The listing builds one solid part. Answer for the finished solid, in the listing's coordinates (mm). A direction names the side the tool comes from. Give positions to 0.01 mm unless a question says otherwise; leave off trailing zeros. Loops run counter-clockwise (first coordinate to the right, second up) from the corner with the lowest first, then second, coordinate; pieces in that order, holes last. Notation, with made-up numbers: M 16.5,27.5 L 27.5,27.5 A17 cw 27.5,38.5 Z; hole C 7,54.25 d7. An arc over 180 degrees is marked long. Return JSON: item names as keys, results as strings.
from build123d import *

# Parameters (mm, degrees)
SKIZZE1_W                            = 42
SKIZZE1_H                            = 25
AUFSATZ_LINEAR_AUSTRAGEN1_DEPTH      = 25
SKIZZE2_W                            = 21
SKIZZE2_H                            = 21
SCHNITT_LINEAR_AUSTRAGEN1_DEPTH      = 43
SCHNITT_LINEAR_AUSTRAGEN2_DEPTH      = 5
SKIZZE4_W                            = 8.8
SKIZZE4_H                            = 21.963947762
AUFSATZ_LINEAR_AUSTRAGEN2_DEPTH      = 21
SCHNITT_LINEAR_AUSTRAGEN3_REACH      = 27
SCHNITT_LINEAR_AUSTRAGEN4_DEPTH      = 5
DURCHGANGSLOCH_F_R_M241_D            = 27
DURCHGANGSLOCH_F_R_M241_DEPTH        = 4
F_5_5_5_5_DURCHMESSER_BOHRUNG1_D     = 5.5
F_5_5_5_5_DURCHMESSER_BOHRUNG1_DEPTH = 25
FASE1_SIZE                           = 2
VERRUNDUNG1_R                        = 1.6
VERRUNDUNG2_R                        = 2
VERRUNDUNG3_R                        = 4
VERRUNDUNG4_R                        = 5.6


with BuildPart() as part:
    # Skizze1 → Aufsatz-Linear austragen1 (new body)
    with BuildSketch(Plane(origin=(25, 0, 0), x_dir=(0, 0, -1), z_dir=(1, 0, 0))):
        with Locations((0, 12.5)):
            Rectangle(SKIZZE1_W, SKIZZE1_H)
    extrude(amount=-AUFSATZ_LINEAR_AUSTRAGEN1_DEPTH)

    # Skizze2 → Schnitt-Linear austragen1 (cut, through all)
    with BuildSketch(Plane.XY.offset(21)):
        with Locations((14.5, 14.5)):
            Rectangle(SKIZZE2_W, SKIZZE2_H)
    extrude(amount=-SCHNITT_LINEAR_AUSTRAGEN1_DEPTH, mode=Mode.SUBTRACT)

    # Skizze3 → Schnitt-Linear austragen2 (cut, through all)
    with BuildSketch(Plane(origin=(4, 0, 0), x_dir=(0, 0, -1), z_dir=(1, 0, 0))):
        with BuildLine():
            Line((-21, 25), (-21, 5.6))
            ThreePointArc((-21, 5.6), (-17.5737339, 15.012569088), (-16.807587704, 25))
            Line((-16.807587704, 25), (-21, 25))
        make_face()
    extrude(amount=-SCHNITT_LINEAR_AUSTRAGEN2_DEPTH, mode=Mode.SUBTRACT)

    # Skizze4 → Aufsatz-Linear austragen2 (add)
    with BuildSketch(Plane(origin=(0, 4, 0), x_dir=(-1, 0, 0), z_dir=(0, 1, 0))):
        with Locations((-20.6, 0)):
            Rectangle(SKIZZE4_W, SKIZZE4_H)
    extrude(amount=AUFSATZ_LINEAR_AUSTRAGEN2_DEPTH)

    # Skizze5 → Schnitt-Linear austragen3 (cut, up to next)
    with BuildSketch(Plane(origin=(25, 0, 0), x_dir=(0, 0, -1), z_dir=(1, 0, 0)), mode=Mode.PRIVATE) as schnitt_linear_austragen3_sk1:
        with BuildLine():
            Line((5, 25), (-5, 25))
            Line((-5, 25), (-5, 12.560423389))
            ThreePointArc((-5, 12.560423389), (0, 7.560423389), (5, 12.560423389))
            Line((5, 12.560423389), (5, 25))
        make_face()
    schnitt_linear_austragen3_tool1 = extrude(schnitt_linear_austragen3_sk1.sketch, amount=-SCHNITT_LINEAR_AUSTRAGEN3_REACH, mode=Mode.PRIVATE) & part.part
    add(schnitt_linear_austragen3_tool1.solids().sort_by_distance((25, 16.778669, 0))[0], mode=Mode.SUBTRACT)

    # Skizze6 → Schnitt-Linear austragen4 (cut, through all)
    with BuildSketch(Plane(origin=(4, 0, 0), x_dir=(0, 0, -1), z_dir=(1, 0, 0))):
        with BuildLine():
            Line((21, 25), (16.807587704, 25))
            ThreePointArc((16.807587704, 25), (17.5737339, 15.012569088), (21, 5.6))
            Line((21, 5.6), (21, 25))
        make_face()
    extrude(amount=-SCHNITT_LINEAR_AUSTRAGEN4_DEPTH, mode=Mode.SUBTRACT)

    # Durchgangsloch für M241
    with Locations(Plane(origin=(4, 0, 0), x_dir=(0, 0, -1), z_dir=(1, 0, 0))):
        with Locations((0, 20)):
            Hole(DURCHGANGSLOCH_F_R_M241_D / 2, depth=DURCHGANGSLOCH_F_R_M241_DEPTH)

    # Ø5.5 (5.5) Durchmesser Bohrung1
    with Locations(Plane(origin=(0, 0, 0), x_dir=(-1, 0, 0), z_dir=(0, -1, 0))):
        with Locations((-14, -16), (-14, 16)):
            Hole(F_5_5_5_5_DURCHMESSER_BOHRUNG1_D / 2, depth=F_5_5_5_5_DURCHMESSER_BOHRUNG1_DEPTH)

    # Fase1
    fase1_edges = [part.edges().sort_by_distance(p)[0] for p in [
        (16.2, 14.5, -10.981973881),
        (16.2, 14.5, 10.981973881),
    ]]
    chamfer(fase1_edges, length=FASE1_SIZE)

    # Verrundung1
    verrundung1_edges = [part.edges().sort_by_distance(p)[0] for p in [
        (4, 4, 0),
    ]]
    fillet(verrundung1_edges, radius=VERRUNDUNG1_R)

    # Verrundung2
    verrundung2_edges = [part.edges().sort_by_distance(p)[0] for p in [
        (21.6, 25, 10.981973881),
        (21.6, 25, -10.981973881),
    ]]
    fillet(verrundung2_edges, radius=VERRUNDUNG2_R)

    # Verrundung3
    verrundung3_edges = [part.edges().sort_by_distance(p)[0] for p in [
        (2, 25, 16.807587704),
        (2, 25, -16.807587704),
    ]]
    fillet(verrundung3_edges, radius=VERRUNDUNG3_R)

    # Verrundung4
    verrundung4_edges = [part.edges().sort_by_distance(p)[0] for p in [
        (0, 0, 0),
    ]]
    fillet(verrundung4_edges, radius=VERRUNDUNG4_R)


solid = part.part
(1) The part is cut by section A-A (x = 14). Determine the outline of the cut face in (y, z).
Values follow:
{"outline": "M 0,-21 L 4,-21 L 4,-18.75 L 0,-18.75 Z; M 0,-13.25 L 4,-13.25 L 4,13.25 L 0,13.25 Z; M 0,18.75 L 4,18.75 L 4,21 L 0,21 Z"}
(2) Straight lines are drawn through the part: line 1 along Z through (x, y) = (14, 1.1); line 2 along Z through (x, y) = (12.5, 3.25); line 3 along X through (y, z) = (22.25, -16). For each, find the intervals that lie inside material, in ascending order.
Values follow:
{"line 1": "-21 to -18.75, -13.25 to 13.25, 18.75 to 21", "line 2": "-21 to -18.3, -13.7 to 13.7, 18.3 to 21", "line 3": "0 to 4"}
(3) Given pin 1 (5.5 mm diameter, centred on x = 22.5, y = 10.5, fed in from -Z); pin 2 (3.5 mm diameter, centred on x = 23, y = 17.5, fed in from +Z); pin 3 (1 mm diameter, centred on x = 3.5, z = 6, fed in from +Y), each flat-ended and moving along its own axis, determine where each tip first touches the part or whether it passes through.
Values follow:
{"pin 1": "z = -10.98", "pin 2": "z = 10.98", "pin 3": "y = 8.17"}
(4) The part is cut by section C-C (z = 17.5). Determine the outline of the cut face in (x, y).
Values follow:
{"outline": "M 0,5.6 A5.6 ccw 5.6,0 L 11.7,0 L 11.7,4 L 5.6,4 A1.6 cw 4,5.6 L 4,15.36 L 0,15.36 Z; M 16.3,0 L 25,0 L 25,4 L 16.3,4 Z"}
(5) A tool of negligible diameter and unlimited length cuts with its end or side. For faces 1 (the flat face through (17.19, 14.35, 9.97)), 2 (the flat face through (17.19, 14.35, -9.97)), 3 (the flat face through (21, 19, 5)), 4 (the cylindrical face through (2.028, 13.264, -17.996)), from which of +Z, -Z, +X, -X, +Y, -Y can it reach the whole face along a straight path? Write none if from no direction.
Values follow:
{"face 1": "+Z, +Y", "face 2": "-Z, +Y", "face 3": "+X, -X, +Y", "face 4": "-Z, +X, -X, +Y"}
(6) Determine the mould class of faces 5 (the cylindrical face through (1.972, 6.505, -0.369)), 6 (the flat face through (13, 4, 0)), 7 (the flat face through (16.2, 7, 0)) for opening direction Y: released by +Y, released by -Y, zero draft, split by the parting line, or undercut.
Values follow:
{"face 5": "undercut", "face 6": "released by +Y", "face 7": "zero draft"}
(7) The part is cut by section B-B (x = 20.75). Determine the outline of the cut face in (y, z).
Values follow:
{"outline": "M 0,-21 L 4,-21 L 4,-10.98 L 23,-10.98 A2 ccw 25,-8.98 L 25,-5 L 12.56,-5 A5 cw 12.56,5 L 25,5 L 25,8.98 A2 ccw 23,10.98 L 4,10.98 L 4,21 L 0,21 Z"}
(8) The part is cut by section D-D (y = 20.5). Determine the outline of the cut face in (x, z).
Values follow:
{"outline": "M 0,-16.81 L 4,-16.81 L 4,-13.49 L 0,-13.49 Z; M 0,13.49 L 4,13.49 L 4,16.81 L 0,16.81 Z; M 16.2,-8.98 L 18.2,-10.98 L 25,-10.98 L 25,-5 L 16.2,-5 Z; M 16.2,5 L 25,5 L 25,10.98 L 18.2,10.98 L 16.2,8.98 Z"}
